Can you work these out from the model? Positions are in its coordinate system, mm. A direction names the side the tool comes from. Coordinates: 2 decimals unless noted, no trailing zeros. Loops run counter-clockwise (first coordinate to the right, second up) from the corner with the lowest first, then second, coordinate; pieces in that order, holes last. Notation, with made-up numbers: (66.5, -26.75) -> (119.5, -26.75) arc R12 cw to (119.5, -20.75) -> close; hole circle Ø7 at (40.25, -37.5). An arc over 180 degrees is marked (long way). Use one line per item in the form item = value. Start each with the question number.
(1) I'm going to push flat-ended pins straight in: pin 1 (1 mm diameter, centred on x = 492.5, y = 20.5, fed in from -Z); pin 2 (1.5 mm diameter, centred on x = 127.5, z = -1.5, fed in from -Y); pin 3 (5 mm diameter, centred on x = 161.5, y = 11, fed in from -Z). Where does each tip first touch, or does it pass through?
(2) Thinking about a two-plate mould opening in Y: for faces 4 (the cylindrical face through (258.37, 2.4, 27.4)), 5 (the conical face through (612.33, 0.42, 16.03)), 6 (the flat face through (871.5, 34, 0)), 7 (the cylindrical face through (2.774, 34.168, -7.587)), which applies, released by +Y, released by -Y, zero draft, split by the parting line, or undercut?
(3) On a 3-axis mill with a long thin cutter (end or side, diameter ignored), from which of +Z, -Z, +X, -X, +Y, -Y can I reach the whole of each face in a straight line? I mean faces 1 (the cylindrical face through (870.2, 29.7, 15.5)), 2 (the flat face through (876, 0, 7)), 3 (the cylindrical face through (619, 0, 27)). Say none if no direction works.
(4) Imagine slicing it at A-A (x = 741). List the corners of the cut face in (y, z) for me.
(5) I need wall thicknesses on line 1 (X direction, y = 0, z = 31.75); line 2 (X direction, y = -16, z = 30); line 3 (Y direction, x = 853.5, z = 0). Which ranges of each line are inside material? Lowest first, please. Write a range as [from, to].
```python
from build123d import *

# Parameters (mm, degrees)
HOLE_WIZARD_16_0_16_2_D     = 16
HOLE_WIZARD_16_0_16_2_DEPTH = 15
HOLE_WIZARD_16_0_16_2_TIP   = 4.806884952
HOLE_WIZARD_M14_1_D         = 12
HOLE_WIZARD_M14_1_DEPTH     = 30
HOLE_WIZARD_M14_1_TIP       = 3.605163714
CHAMFER_1_SIZE              = 1


with BuildPart() as part:
    # 草图1 → 旋转1 (revolve)
    with BuildSketch(Plane.XY, mode=Mode.PRIVATE) as revolve_1_sk:
        Polygon((0, 0), (0, 35), (4.5, 35), (4.5, 33.5), (7.2, 33.5), (7.2, 35), (868.8, 35), (868.8, 33.5), (871.5, 33.5), (871.5, 35), (876, 35), (876, 0), align=None)
    revolve(revolve_1_sk.sketch.rotate(Axis((0, 0, 0), (1, 0, 0)), 90), axis=Axis((0, 0, 0), (1, 0, 0)))

    # Ø16.0 (16) 直径孔2
    with Locations(Plane.XY.offset(35)):
        with Locations((266, 0), (611, 0)):
            Hole(HOLE_WIZARD_16_0_16_2_D / 2, depth=HOLE_WIZARD_16_0_16_2_DEPTH)
            with Locations((0, 0, -(HOLE_WIZARD_16_0_16_2_DEPTH + HOLE_WIZARD_16_0_16_2_TIP / 2))):  # 118° drill point
                Cone(0, HOLE_WIZARD_16_0_16_2_D / 2, HOLE_WIZARD_16_0_16_2_TIP, mode=Mode.SUBTRACT)

    # M14 螺纹孔1
    with Locations(Plane(origin=(876, 0, 0), x_dir=(0, 0, 1), z_dir=(1, 0, 0))):
        with Locations((0, 0)):
            Hole(HOLE_WIZARD_M14_1_D / 2, depth=HOLE_WIZARD_M14_1_DEPTH)
            with Locations((0, 0, -(HOLE_WIZARD_M14_1_DEPTH + HOLE_WIZARD_M14_1_TIP / 2))):  # 118° drill point
                Cone(0, HOLE_WIZARD_M14_1_D / 2, HOLE_WIZARD_M14_1_TIP, mode=Mode.SUBTRACT)

    # 倒角1
    chamfer_1_edges = [part.edges().sort_by_distance(p)[0] for p in [
        (0, 0, -35),
        (876, 0, -35),
    ]]
    chamfer(chamfer_1_edges, length=CHAMFER_1_SIZE)


solid = part.part
```
Worked out:
q1.pin_1 = -28.72
q1.pin_2 = -34.99
q1.pin_3 = -33.95
q2.face_4 = undercut
q2.face_5 = undercut
q2.face_6 = zero draft
q2.face_7 = split by the parting line
q3.face_1 = none
q3.face_2 = +Z, -Z, +X, +Y, -Y
q3.face_3 = +Z
q4.outline = circle Ø70 at (0, 0)
q5.line_1 = [0, 258], [274, 603], [619, 876]
q5.line_2 = [0, 4.5], [7.2, 868.8], [871.5, 876]
q5.line_3 = [-35, -6], [6, 35]
